Drawing for the job (mm, zero at the part's lowest x, y, z). A direction names the side the tool comes from. Coordinates: 2 decimals unless noted, no trailing zeros. Write each loop counter-clockwise with the first axis right and the second up, starting at its lowest first coordinate (ties: lowest second). Pieces come first, ordered by that corner, then holes. Notation, with made-up numbers: M -15.75,51.5 L -10.75,51.5 A29 ccw -10.75,76.5 Z; hole C 26,9.25 d3. An arc over 180 degrees is marked long. Put each result on its own line as item: value. Start each with the question number.
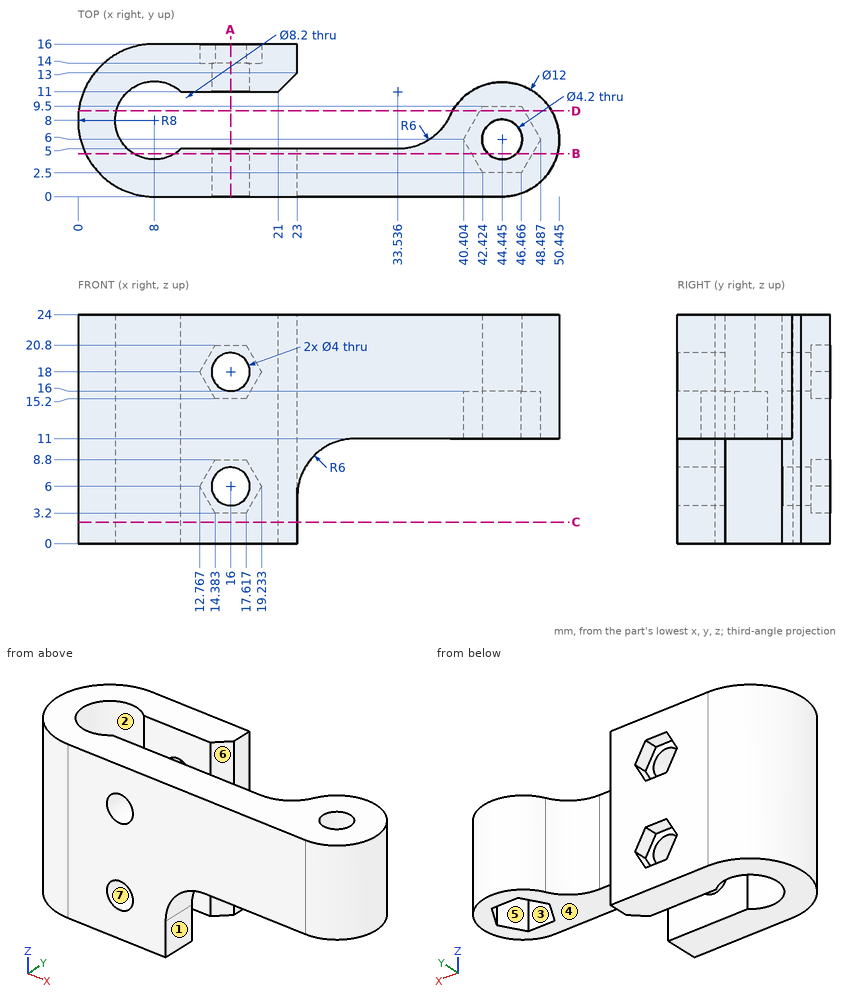
(1) Drop flat-ended pins along their axis: pin 1 (1.6 mm diameter, centred on x = 17, y = 15.5, fed in from -Z); pin 2 (2 mm diameter, centred on x = 45.5, y = 4.5, fed in from -Z); pin 3 (1.5 mm diameter, centred on y = 2, z = 2, fed in from +X); pin 4 (1 mm diameter, centred on y = 4.5, z = 11, fed in from +X). Give the stop position or say it passes through.
(2) Slice it at A-A, the plane x = 16. State how many separate pieces and enclosed holes the cut face has.
(3) Which spindle directions (+Z, -Z, +X, -X, +Y, -Y) get a long thin tool onto all of the face, cutting with end or side? Do the marked faces 5, 6 and 7. Say none if no direction does.
(4) Slice it at B-B, the plane y = 4.5. Write the cut outline in (x, z) (1 decimal).
(5) Drill centre lines: line 1 (Z direction, x = 16, y = 3.8); line 2 (Y direction, x = 13, z = 12.5); line 3 (X direction, y = 8, z = 12.5). Where is each one in solid material? Low to high. Write a range as [from, to].
(6) Slice it at D-D, the plane y = 9. Write the cut outline in (x, z) (1 decimal).
(7) Slice it at C-C, the plane z = 2.25. Write the cut outline in (x, y) (1 decimal).
(8) Two-plate mould, pull along X, no slides. Class the marked faces 1, 2, 3 and 4: +X half, -X half, draft (parallel to the pull), parting line (faces both ways), or undercut.
Result set:
1. pin 1: stops at z = 0
1. pin 2: stops at z = 16
1. pin 3: stops at x = 23
1. pin 4: stops at x = 50.36
2. separate pieces: 6
2. enclosed holes: 0
3. face 5: -Z
3. face 6: +Z, -Z
3. face 7: +Y, -Y
4. outline: M 0.8,0 L 5.9,0 L 5.9,24 L 0.8,24 Z; M 10.1,0 L 23,0 L 23,5 A6 cw 29,11 L 41.3,11 L 41.3,16 L 43,16 L 43,24 L 10.1,24 Z; M 45.9,16 L 47.6,16 L 47.6,11 L 50.3,11 L 50.3,24 L 45.9,24 Z; hole C 16,6 d4; hole C 16,18 d4
5. line 1: z = [0, 4], [8, 16], [20, 24]
5. line 2: y = [0, 5], [11, 16]
5. line 3: x = [0, 3.9], [38.73, 41.56], [47.33, 50.1]
6. outline: M 0.1,0 L 4,0 L 4,24 L 0.1,24 Z; M 39.2,11 L 42.1,11 L 42.1,16 L 46.8,16 L 46.8,11 L 49.6,11 L 49.6,24 L 39.2,24 Z
7. outline: M 8,0 L 23,0 L 23,5 L 10.8,5 A4.1 cw long 10.8,11 L 21,11 L 23,13 L 23,16 L 8,16 A8 ccw Z
8. face 1: +X half
8. face 2: undercut
8. face 3: undercut
8. face 4: draft
